```python
from build123d import *

# Parameters (mm, degrees)
BOSS_EXTRUDE1_DEPTH = 381
CUT_EXTRUDE1_REACH  = 383.687
SKETCH2_R           = 3.175
SKETCH3_R           = 2.54
CUT_EXTRUDE2_DEPTH  = 7.62
CUT_EXTRUDE3_START  = -7.62
SKETCH4_R           = 2.54
CUT_EXTRUDE3_DEPTH  = 7.62
SKETCH5_W           = 6.35
SKETCH5_H           = 6.35
CUT_EXTRUDE4_DEPTH  = 345.44
SKETCH7_W           = 345.44
SKETCH7_H           = 19.05
CUT_EXTRUDE5_DEPTH  = 382.528799699


with BuildPart() as part:
    # Sketch1 → Boss-Extrude1 (new body)
    with BuildSketch(Plane.XY):
        Polygon((0, 0), (-12.7, 0), (-12.7, 19.05), (-6.35, 19.05), (-6.35, 6.35), (0, 6.35), align=None)
    extrude(amount=-BOSS_EXTRUDE1_DEPTH)

    # Sketch2 → Cut-Extrude1 (cut, up to next)
    with BuildSketch(Plane.ZY.offset(12.7), mode=Mode.PRIVATE) as cut_extrude1_sk1:
        with Locations(Location((-365.76, 12.065, 0), (0, 0, 270))):
            Circle(SKETCH2_R)
    cut_extrude1_tool1 = extrude(cut_extrude1_sk1.sketch, amount=-CUT_EXTRUDE1_REACH, mode=Mode.PRIVATE) & part.part
    add(cut_extrude1_tool1.solids().sort_by_distance((-12.7, 12.065, -365.76))[0], mode=Mode.SUBTRACT)

    # Sketch3 → Cut-Extrude2 (cut)
    with BuildSketch(Plane(origin=(0, 19.05, 0), x_dir=(1, 0, 0), z_dir=(0, 1, 0))):
        with Locations(Location((-9.525, 6.35, 0), (0, 0, 270))):
            Circle(SKETCH3_R)
        with Locations(Location((-9.525, 374.65, 0), (0, 0, 270))):
            Circle(SKETCH3_R)
    extrude(amount=-CUT_EXTRUDE2_DEPTH, mode=Mode.SUBTRACT)

    # Sketch4 → Cut-Extrude3 (cut)
    with BuildSketch(Plane.XZ.offset(CUT_EXTRUDE3_START)):
        with Locations(Location((-9.525, -374.65, 0), (0, 0, 90))):
            Circle(SKETCH4_R)
        with Locations(Location((-9.525, -6.35, 0), (0, 0, 90))):
            Circle(SKETCH4_R)
    extrude(amount=CUT_EXTRUDE3_DEPTH, mode=Mode.SUBTRACT)

    # Sketch5 → Cut-Extrude4 (cut)
    with BuildSketch(Plane(origin=(0, 0, -381), x_dir=(-1, 0, 0), z_dir=(0, 0, -1))):
        with Locations((3.175, 3.175)):
            Rectangle(SKETCH5_W, SKETCH5_H)
    extrude(amount=-CUT_EXTRUDE4_DEPTH, mode=Mode.SUBTRACT)

    # Sketch7 → Cut-Extrude5 (cut, through all)
    with BuildSketch(Plane(origin=(-6.35, 0, 0), x_dir=(0, 0, -1), z_dir=(1, 0, 0))):
        with Locations((208.28, 9.525)):
            Rectangle(SKETCH7_W, SKETCH7_H)
    extrude(amount=-CUT_EXTRUDE5_DEPTH, mode=Mode.SUBTRACT)


solid = part.part
```
Source: CAD feature listing. Evaluate the final solid. Frame: model axes, mm. A direction names the side the tool comes from. Coordinates: 2 decimals unless noted, no trailing zeros. Write each loop counter-clockwise with the first axis right and the second up, starting at its lowest first coordinate (ties: lowest second). Pieces come first, ordered by that corner, then holes. Notation, with made-up numbers: M -12.5,0 L 26.5,0 A8 ccw 26.5,11 Z; hole C -38,64 d9. An arc over 180 degrees is marked long. Answer as a JSON object with one key per item and string values.
1. Cut plane D-D on z = -28.5. Output: boundary loops of the cut face in (x, y).
Evaluation:
{"outline": "M -12.7,0 L 0,0 L 0,6.35 L -6.35,6.35 L -6.35,19.05 L -12.7,19.05 Z"}
2. Contact query for flat-ended pins moving along their axis: P1, Ø1.5, axis at x = -9.5, z = -5.5, coming from the -Y side; P2, Ø1.5, axis at x = -3, z = -17.5, coming from the +Y side; P3, Ø6, axis at y = 11.5, z = -28.5, coming from the +X side. Output: stop coordinate, or through.
Evaluation:
{"P1": "y = 7.62", "P2": "y = 6.35", "P3": "x = -6.35"}
3. Draft query along Z for faces 4 (the flat face through (-9, 11.43, -6)), 5 (the flat face through (-8, 8, 0)), 6 (the cylindrical face through (-12.005, 15.293, -6.901)), 7 (the flat face through (-12.7, 9, -18)). Return one class per face: released by +Z, released by -Z, zero draft, split by the parting line, or undercut.
Evaluation:
{"face 4": "undercut", "face 5": "released by +Z", "face 6": "undercut", "face 7": "zero draft"}
4. Cut plane B-B on y = 2.75. Output: boundary loops of the cut face in (x, z) (3 decimals), plus the area to 3 significant figures.
Evaluation:
{"outline": "M -12.7,-35.56 L 0,-35.56 L 0,0 L -12.7,0 Z; hole C -9.525,-6.35 d5.08", "area": "431 mm^2"}
5. Cut plane A-A on z = -6.35. Output: boundary loops of the cut face in (x, y) (3 decimals), plus the area to 3 significant figures.
Evaluation:
{"outline": "M -12.7,0 L -12.065,0 L -12.065,7.62 L -6.985,7.62 L -6.985,0 L 0,0 L 0,6.35 L -6.35,6.35 L -6.35,19.05 L -6.985,19.05 L -6.985,11.43 L -12.065,11.43 L -12.065,19.05 L -12.7,19.05 Z", "area": "83.9 mm^2"}
6. Ray query, L1, parallel to X at y = 17.25, z = -6.35 (3 decimals); L2, parallel to X at y = 2, z = -6.35 (3 decimals); L3, parallel to Z at x = -9.25, y = 13. Return the intervals inside material, ascending.
Evaluation:
{"L1": "-12.7 to -12.065, -6.985 to -6.35", "L2": "-12.7 to -12.065, -6.985 to 0", "L3": "-35.56 to -8.88, -3.82 to 0"}
7. Access query for faces 1 (the flat face through (-6, 0, -18)), 2 (the flat face through (-6.35, 13, -18)), 3 (the flat face through (-10, 7.62, -6)). Directions: +Z, -Z, +X, -X, +Y, -Y. A direction counts if a zero-diameter tool reaches every point of the face in a straight line with its end or side. Return the directions, or none.
Evaluation:
{"face 1": "+Z, -Z, +X, -X, -Y", "face 2": "+Z, -Z, +X, +Y", "face 3": "-Y"}
8. Cut plane C-C on x = -8.5. Output: boundary loops of the cut face in (y, z), plus the area to 3 significant figures.
Evaluation:
{"outline": "M 0,-35.56 L 19.05,-35.56 L 19.05,-8.67 L 11.43,-8.67 L 11.43,-4.03 L 19.05,-4.03 L 19.05,0 L 0,0 L 0,-4.03 L 7.62,-4.03 L 7.62,-8.67 L 0,-8.67 Z", "area": "607 mm^2"}
